Autodesk Inventor part; units mm, degrees
ref_plane "YZ Plane" through (0, 0, 0) normal (1, 0, 0) x (0, 1, 0)
ref_plane "XZ Plane" through (0, 0, 0) normal (0, 1, 0) x (-1, 0, 0)
ref_plane "XY Plane" through (0, 0, 0) normal (0, 0, 1) x (1, 0, 0)
sketch "스케치4" plane through (0, 0, 0) normal (1, 0, 0) x (0, 1, 0)
  line L0 (0, 0) -> (0, 70)
  line L1 (0, 70) -> (20, 70)
  line L2 (20, 70) -> (20, 50)
  line L3 (20, 50) -> (15, 45)
  line L4 (15, 45) -> (15, 25)
  line L5 (15, 25) -> (20, 20)
  line L6 (20, 20) -> (20, 0)
  line L7 (20, 0) -> (0, 0)
  dimension "d98" = 70
  dimension "d99" = 20
  dimension "d100" = 20
  dimension "d101" = 20
  dimension "d102" = 20
  dimension "d103" = 5
  dimension "d104" = 5
revolve "회전2" add sketch "스케치4" angle 360 about axis through (0, 0, 0) along (0, 0, 1)
sketch "스케치5" plane through (0, 0, 70) normal (0, 0, 1) x (1, 0, 0)
  circle A0 centre (0, 0) radius 5
  dimension "d106" = 10
extrude "돌출1" cut sketch "스케치5" against normal blind 20
sketch "스케치6" plane through (0, 0, 50) normal (0, 0, 1) x (1, 0, 0)
  circle A0 centre (0, 0) radius 12.5
  dimension "d109" = 25
extrude "돌출2" cut sketch "스케치6" against normal blind 30
sketch "스케치7" plane through (0, 0, 20) normal (0, 0, 1) x (1, 0, 0)
  circle A0 centre (0, 0) radius 5
  dimension "d112" = 10
extrude "돌출3" cut sketch "스케치7" against normal up to next
properties part number "기본 투상 연습4"
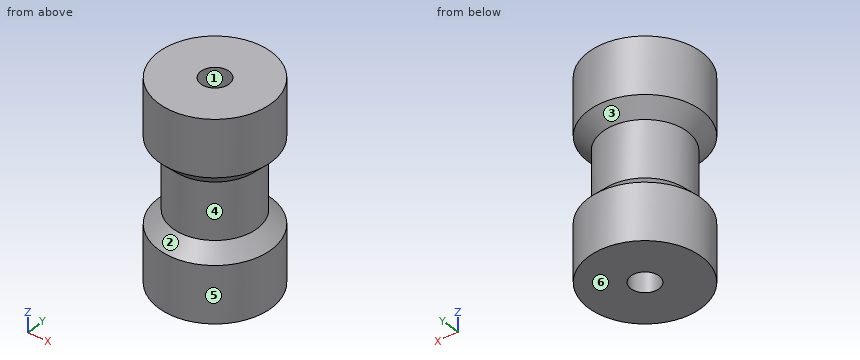
Read the model definition and answer for the solid it produces. Units are mm, in the model's axes. Face numbers are marked on the shaded views. A direction names the side the tool comes from. Give positions to 0.01 mm unless a question says otherwise; leave off trailing zeros. Loops run counter-clockwise (first coordinate to the right, second up) from the corner with the lowest first, then second, coordinate; pieces in that order, holes last.
Item 1: The part is cut by section A-A (x = 0). Write down the section's boundary in (y, z), and give its area (3 significant figures).
Item 2: The part is cut by section D-D (z = 61). Write down the section's boundary in (x, y).
Item 3: The part is cut by section C-C (z = 47.5). Write down the section's boundary in (x, y).
Item 4: Find the intervals of material crossed by line 1 along Z through (x, y) = (1, 11.5); line 2 along Y through (x, z) = (0, 28.25); line 3 along Y through (x, z) = (0, 15.5), in increasing order.
Item 5: The mould has two halves that part along Z. Classify the marked faces 3, 4, 5 and 6: released by +Z, released by -Z, zero draft, split by the parting line, or undercut.
Item 6: For the marked faces 1 and 2, determine the directions among +Z, -Z, +X, -X, +Y, -Y from which every point of the face is accessible in a straight line to the end or side of a thin tool.
Item 7: Each of these flat-tipped pins is pushed along its axis until it touches: pin 1 Ø8 at (y, z) = (5, 36) entering from -X; pin 2 Ø8 at (y, z) = (-5, 62) entering from -X (3 decimals); pin 3 Ø5 at (y, z) = (1, 56.5) entering from +X; pin 4 Ø8 at (x, y) = (0, 0) entering from -Z. Where does it stop, or does it pass through?
Taken from the geometry:
1. outline: (-20, 0) - (-5, 0) - (-5, 20) - (-12.5, 20) - (-12.5, 50) - (-5, 50) - (-5, 70) - (-20, 70) - (-20, 50) - (-15, 45) - (-15, 25) - (-20, 20) - close; (5, 0) - (20, 0) - (20, 20) - (15, 25) - (15, 45) - (20, 50) - (20, 70) - (5, 70) - (5, 50) - (12.5, 50) - (12.5, 20) - (5, 20) - close
1. area: 1,400 mm2
2. outline: circle Ø40 at (0, 0); hole circle Ø10 at (0, 0)
3. outline: circle Ø35 at (0, 0); hole circle Ø25 at (0, 0)
4. line 1: z = 0 to 20, 50 to 70
4. line 2: y = -15 to -12.5, 12.5 to 15
4. line 3: y = -20 to -5, 5 to 20
5. face 3: undercut
5. face 4: undercut
5. face 5: zero draft
5. face 6: released by -Z
6. face 1: +Z, -Z
6. face 2: none
7. pin 1: stops at x = -14.97
7. pin 2: stops at x = -19.975
7. pin 3: stops at x = 20
7. pin 4: passes through
